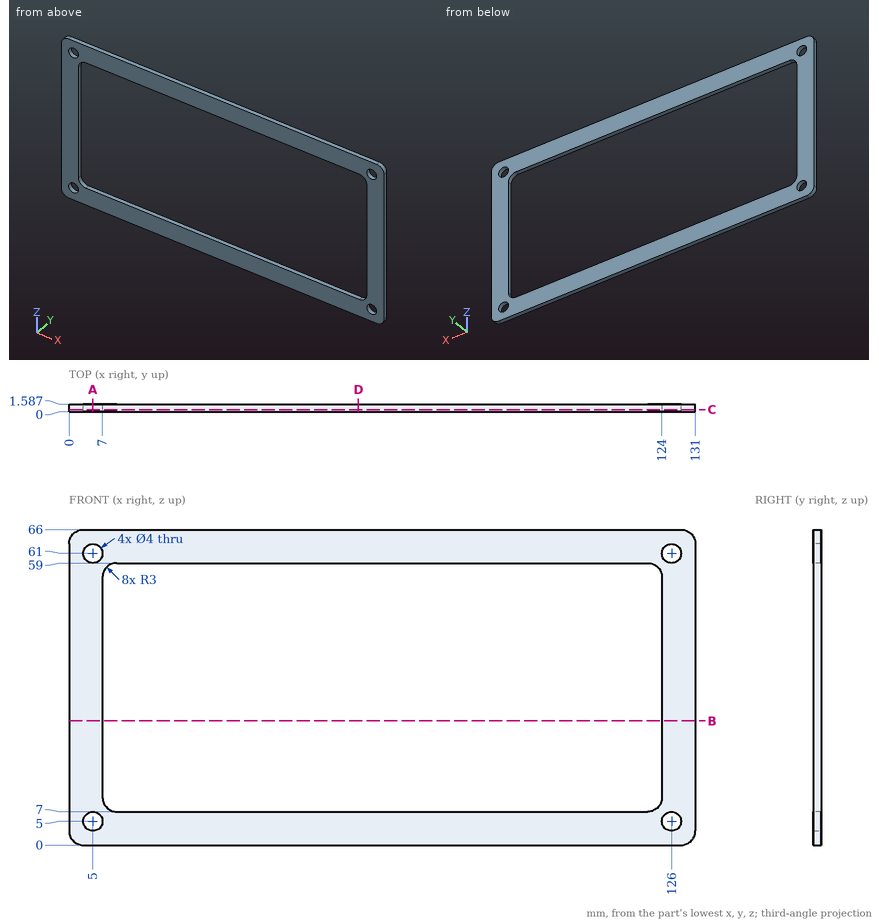
Design review of the part shown in the three views and the two pictorial views. Dimensions are in mm from the part's minimum x, y and z. Give positions to 0.01 mm unless a question says otherwise; leave off trailing zeros. Loops run counter-clockwise (first coordinate to the right, second up) from the corner with the lowest first, then second, coordinate; pieces in that order, holes last. Notation, with made-up numbers: (74, 7) -> (116, 7) arc R23 ccw to (116, 16) -> close; hole circle Ø3 at (35.25, -12). An arc over 180 degrees is marked (long way). Write each question's results on one line, items separated by ' | '.
Q1. Take a section at B-B, the plane z = 26. Write out the cut boundary in (x, y).
Reply:
outline: (0, 0) -> (7, 0) -> (7, 1.59) -> (0, 1.59) -> close; (124, 0) -> (131, 0) -> (131, 1.59) -> (124, 1.59) -> close
Q2. Take a section at D-D, the plane x = 60.5. Write out the cut boundary in (y, z).
Reply:
outline: (0, 0) -> (1.59, 0) -> (1.59, 7) -> (0, 7) -> close; (0, 59) -> (1.59, 59) -> (1.59, 66) -> (0, 66) -> close
Q3. Take a section at A-A, the plane x = 5. Write out the cut boundary in (y, z).
Reply:
outline: (0, 0) -> (1.59, 0) -> (1.59, 3) -> (0, 3) -> close; (0, 7) -> (1.59, 7) -> (1.59, 59) -> (0, 59) -> close; (0, 63) -> (1.59, 63) -> (1.59, 66) -> (0, 66) -> close
Q4. Wall thickness on L1, parallel to X at y = 0.9, z = 61; L2, parallel to Z at x = 90, y = 1.55; L3, parallel to X at y = 0.8, z = 21.5: over which ranges is each line inside the solid? List them lowest first.
Reply:
L1: x = 0 to 3, 7 to 124, 128 to 131 | L2: z = 0 to 7, 59 to 66 | L3: x = 0 to 7, 124 to 131
Q5. Take a section at C-C, the plane y = 0.4. Write out the cut boundary in (x, z), plus the area to 3 significant figures.
Reply:
outline: (0, 3) arc R3 ccw to (3, 0) -> (128, 0) arc R3 ccw to (131, 3) -> (131, 63) arc R3 ccw to (128, 66) -> (3, 66) arc R3 ccw to (0, 63) -> close; hole circle Ø4 at (5, 5); hole circle Ø4 at (5, 61); hole (7, 10) arc R3 ccw to (10, 7) -> (121, 7) arc R3 ccw to (124, 10) -> (124, 56) arc R3 ccw to (121, 59) -> (10, 59) arc R3 ccw to (7, 56) -> close; hole circle Ø4 at (126, 5); hole circle Ø4 at (126, 61) | area: 2,510 mm²
